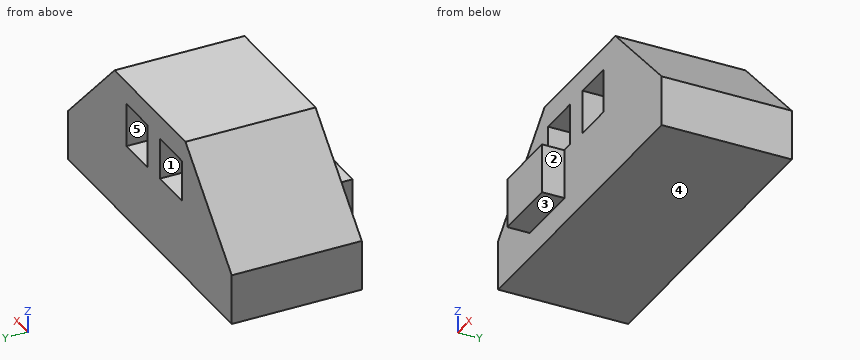
from build123d import *

# Parameters (mm, degrees)
F0_W     = 179.547206
F0_H     = 79.261191
F1_DEPTH = 73.152
F2_SIZE  = 50.8
F3_W     = 24.096457
F3_H     = 23.186842
F4_DEPTH = 286.004
F5_W     = 23.281777
F5_H     = 24.811177
F6_DEPTH = 221.742
F7_SIZE  = 50.8
F8_W     = 38.1
F8_H     = 27.94
F9_DEPTH = 12.7


with BuildPart() as f1:
    # F0 (on Front) → F1 (new body)
    with BuildSketch(Plane.XZ):
        with Locations((5.070895, 8.037225)):
            Rectangle(F0_W, F0_H)
    extrude(amount=F1_DEPTH)

    # F2
    f2_edges = [f1.edges().sort_by_distance(p)[0] for p in [
        (-84.702708, -36.576, 47.66782),
    ]]
    chamfer(f2_edges, length=F2_SIZE)

    # F3 (on face) → F4 (cut)
    with BuildSketch(Plane.XZ.offset(73.152)):
        with Locations((-18.007661, 22.801763)):
            Rectangle(F3_W, F3_H)
    extrude(amount=-F4_DEPTH, mode=Mode.SUBTRACT)

    # F5 (on face) → F6 (cut)
    with BuildSketch(Plane.XZ.offset(73.152)):
        with Locations((19.424999, 22.71818)):
            Rectangle(F5_W, F5_H)
    extrude(amount=-F6_DEPTH, mode=Mode.SUBTRACT)

    # F7
    f7_edges = [f1.edges().sort_by_distance(p)[0] for p in [
        (94.844498, -36.576, 47.66782),
    ]]
    chamfer(f7_edges, length=F7_SIZE)

    # F8 (on face) → F9 (join)
    with BuildSketch(Plane.XZ.offset(73.152)):
        with Locations((-30.878472, -3.178807)):
            Rectangle(F8_W, F8_H)
    extrude(amount=F9_DEPTH)


solid = f1.part
Model file for the job. Use its own axes, mm. Face numbers are marked on the shaded views. A direction names the side the tool comes from. Give positions to 0.01 mm unless a question says otherwise; leave off trailing zeros. Order: outer loops, then holes, each group sorted by start corner. A loop starts at its lowest first (then second) coordinate and runs counter-clockwise, first axis right, second up. Notation, with made-up numbers: (84, 81.25) - (123, 81.25) arc R24 ccw to (123, 99.25) - close; hole circle Ø4 at (19, -34.75). An arc over 180 degrees is marked (long way). Return JSON: item names as keys, results as strings.
1) Cut at D-D, the plane z = 17. Give the cut face in (x, y), plus the area to 3 significant figures.
Geometry says:
{"outline": "(-64.57, -73.15) - (-30.06, -73.15) - (-30.06, 0) - (-64.57, 0) - close; (-5.96, -73.15) - (7.78, -73.15) - (7.78, 0) - (-5.96, 0) - close; (31.07, -73.15) - (74.71, -73.15) - (74.71, 0) - (31.07, 0) - close", "area": "6,720 mm²"}
2) Probe line 1 (X direction, y = -44.5, z = 34); line 2 (Z direction, x = -9, y = -6); line 3 (Z direction, x = 23.5, y = -8). List the from-to ranges inside material, lowest first. Write a range as from..to.
Geometry says:
{"line 1": "-47.57..-30.06, -5.96..7.78, 31.07..57.71", "line 2": "-31.59..11.21, 34.4..47.67", "line 3": "-31.59..10.31, 35.12..47.67"}
3) Cut at C-C, the plane z = -10. Give the cut face in (x, y), plus the area to 3 significant figures.
Geometry says:
{"outline": "(-84.7, -73.15) - (-49.93, -73.15) - (-49.93, -85.85) - (-11.83, -85.85) - (-11.83, -73.15) - (94.84, -73.15) - (94.84, 0) - (-84.7, 0) - close", "area": "13,600 mm²"}
4) Flat gauge pins, fed straight in: P1, Ø4, axis at x = -32, y = -82.5, coming from the +Z side; P2, Ø18.5, axis at y = -44, z = 18, coming from the +X side; P3, Ø2, axis at y = -21, z = 34, coming from the +X side. Where does each tip first touch, or does it go through?
Geometry says:
{"P1": "z = 10.79", "P2": "x = 82.96", "P3": "x = 58.71"}
5) Cut at A-A, the plane x = 17. Give the cut face in (y, z), plus the area to 3 significant figures.
Geometry says:
{"outline": "(-73.15, -31.59) - (0, -31.59) - (0, 10.31) - (-73.15, 10.31) - close; (-73.15, 35.12) - (0, 35.12) - (0, 47.67) - (-73.15, 47.67) - close", "area": "3,980 mm²"}
6) Cut at B-B, the plane y = -44.5. Give the cut face in (x, z), plus the area to 3 significant figures.
Geometry says:
{"outline": "(-84.7, -31.59) - (94.84, -31.59) - (94.84, -3.13) - (44.04, 47.67) - (-33.9, 47.67) - (-84.7, -3.13) - close; hole (-30.06, 11.21) - (-5.96, 11.21) - (-5.96, 34.4) - (-30.06, 34.4) - close; hole (7.78, 10.31) - (31.07, 10.31) - (31.07, 35.12) - (7.78, 35.12) - close", "area": "10,500 mm²"}
7) Pull direction Z, two halves, no side cores. Call the marked faces 1, 2 and 3: pulls with the +Z half, pulls with the -Z half, needs draft (parallel to the pull), parting line crosses it, or undercut.
Geometry says:
{"face 1": "undercut", "face 2": "needs draft", "face 3": "pulls with the -Z half"}
8) 3-axis set-ups, long thin cutter, end or side, ignore diameter. For the marked faces 4 and 5: which of +Z, -Z, +X, -X, +Y, -Y reach the whole face in a straight line?
Geometry says:
{"face 4": "-Z, +X, -X, +Y, -Y", "face 5": "+Y, -Y"}
